For this review, take the finished solid that the model builds, in its own axes (mm). A direction names the side the tool comes from. Give positions to 0.01 mm unless a question says otherwise; leave off trailing zeros. Loops run counter-clockwise (first coordinate to the right, second up) from the corner with the lowest first, then second, coordinate; pieces in that order, holes last. Notation, with made-up numbers: (31.25, 42) -> (52.25, 42) arc R18 cw to (52.25, 49) -> close; hole circle Ø9 at (4.25, -7). An arc over 180 degrees is marked (long way). Answer as CSV lines item,"result". Start each with the question number.
Item 1: Add section A-A on x = 16.2. State the section outline as (y, z) points.
Item 2: Machinability: for faces 5 (the face through (12, 0, 1)), 6 (the face through (16.447, 0.546, 48.118)), which of the approach directions +Z, -Z, +X, -X, +Y, -Y give a long, thin tool a straight path to every point of the face, cutting with its end or side? Answer none if there is none.
Item 3: Add section C-C on x = 6.5. State the section outline as (y, z) points.
Item 4: For L1, parallel to Z at x = 16.2, y = 0.7; L2, parallel to Y at x = 20.5, z = -24.5; L3, parallel to Y at x = -10, z = 38, list the stretches that pass through material, from the lowest coordinate up. Write a range as from..to.
Item 5: Clearance check with flat-ended pins moving along their axes: P1, Ø2.5, axis at x = 16.2, z = 50, coming from the +Y side; P2, Ø3, axis at x = -14, z = 20.5, coming from the -Y side; P3, Ø20, axis at x = 14, z = 34, coming from the -Y side; P4, Ø4, axis at y = -7, z = 38, coming from the +X side. State where each tip first meets the part, or that it passes through.
Item 6: Add section B-B on z = 0. State the section outline as (x, y) points.
Item 7: Add section D-D on y = -2. State the section outline as (x, z) points, plus the area to 3 significant figures.
Item 8: The part is to be moulded in two halves that separate along X. For faces 1 (the face through (18.097, 0.546, -0.083)), 2 (the face through (25, 1, 1)), 3 (the face through (-13.612, -4.395, 1.05)), 4 (the face through (18.097, 0.546, -50.083)), say which applies: +X half, -X half, draft (parallel to the pull), parting line (faces both ways), or undercut.
```python
from build123d import *

# Parameters (mm, degrees)
SALIENTE_EXTRUIR1_DEPTH                              = 75
AVELLANADO_PARA_TORNILLO_CON_CABEZA_OVAL_D           = 3.7973
AVELLANADO_PARA_TORNILLO_CON_CABEZA_OVAL_DEPTH       = 20
AVELLANADO_PARA_TORNILLO_CON_CABEZA_OVAL_CSINK_D     = 7.0866
AVELLANADO_PARA_TORNILLO_CON_CABEZA_OVAL_CSINK_ANGLE = 82
AVELLANADO_PARA_TORNILLO_CON_CABEZA_OVAL_TIP         = 1.140824014


with BuildPart() as part:
    # Croquis1 → Saliente-Extruir1 (new body, symmetric)
    with BuildSketch(Plane.XY):
        Polygon((25, 0), (25, 3), (-0.803847577, 3), (-26.784609691, -12), (-20.784609691, -12), (0, 0), align=None)
    extrude(amount=SALIENTE_EXTRUIR1_DEPTH, both=True)

    # Avellanado para tornillo con cabeza ovalada de #61
    with Locations(Plane(origin=(16.2, 3, -50), x_dir=(1, 0, 0), z_dir=(0, 1, 0))):
        with Locations((0, 0), (0, -50), (0, -100)):
            CounterSinkHole(AVELLANADO_PARA_TORNILLO_CON_CABEZA_OVAL_D / 2, AVELLANADO_PARA_TORNILLO_CON_CABEZA_OVAL_CSINK_D / 2, depth=AVELLANADO_PARA_TORNILLO_CON_CABEZA_OVAL_DEPTH, counter_sink_angle=AVELLANADO_PARA_TORNILLO_CON_CABEZA_OVAL_CSINK_ANGLE)
            with Locations((0, 0, -(AVELLANADO_PARA_TORNILLO_CON_CABEZA_OVAL_DEPTH + AVELLANADO_PARA_TORNILLO_CON_CABEZA_OVAL_TIP / 2))):  # 118° drill point
                Cone(0, AVELLANADO_PARA_TORNILLO_CON_CABEZA_OVAL_D / 2, AVELLANADO_PARA_TORNILLO_CON_CABEZA_OVAL_TIP, mode=Mode.SUBTRACT)


solid = part.part
```
Computed values:
1,outline,"(0, -75) -> (3, -75) -> (3, -53.54) -> (1.11, -51.9) -> (0, -51.9) -> close; (0, -48.1) -> (1.11, -48.1) -> (3, -46.46) -> (3, -3.54) -> (1.11, -1.9) -> (0, -1.9) -> close; (0, 1.9) -> (1.11, 1.9) -> (3, 3.54) -> (3, 46.46) -> (1.11, 48.1) -> (0, 48.1) -> close; (0, 51.9) -> (1.11, 51.9) -> (3, 53.54) -> (3, 75) -> (0, 75) -> close"
2,face 5,"+Z, -Z, +X, -Y"
2,face 6,"+Y, -Y"
3,outline,"(0, -75) -> (3, -75) -> (3, 75) -> (0, 75) -> close"
4,L1,"-75..-51.9, -48.1..-1.9, 1.9..48.1, 51.9..75"
4,L2,"0..3"
4,L3,"-5.77..-2.31"
5,P1,"through"
5,P2,"y = -8.95"
5,P3,"y = 0"
5,P4,"x = -8.66"
6,outline,"(-26.78, -12) -> (-20.78, -12) -> (0, 0) -> (14.3, 0) -> (14.3, 1.11) -> (12.66, 3) -> (-0.8, 3) -> close; (18.1, 0) -> (25, 0) -> (25, 3) -> (19.74, 3) -> (18.1, 1.11) -> close"
7,outline,"(-9.46, -75) -> (-3.46, -75) -> (-3.46, 75) -> (-9.46, 75) -> close"
7,area,"900 mm²"
8,face 1,"undercut"
8,face 2,"+X half"
8,face 3,"-X half"
8,face 4,"undercut"
